Source: three-view drawing plus pictorial views. Frame: mm from the lowest corner of the part. A direction names the side the tool comes from. Round coordinates to 2 decimals unless told otherwise and drop trailing zeros. Write each loop counter-clockwise with the first axis right and the second up, starting at its lowest first coordinate (ties: lowest second). Pieces come first, ordered by that corner, then holes. Notation, with made-up numbers: (66.25, 66.25) -> (99.25, 66.25) arc R14 cw to (99.25, 74.25) -> close; hole circle Ø8 at (13, -12.5). An arc over 180 degrees is marked (long way). Put each result on its own line as item: value.
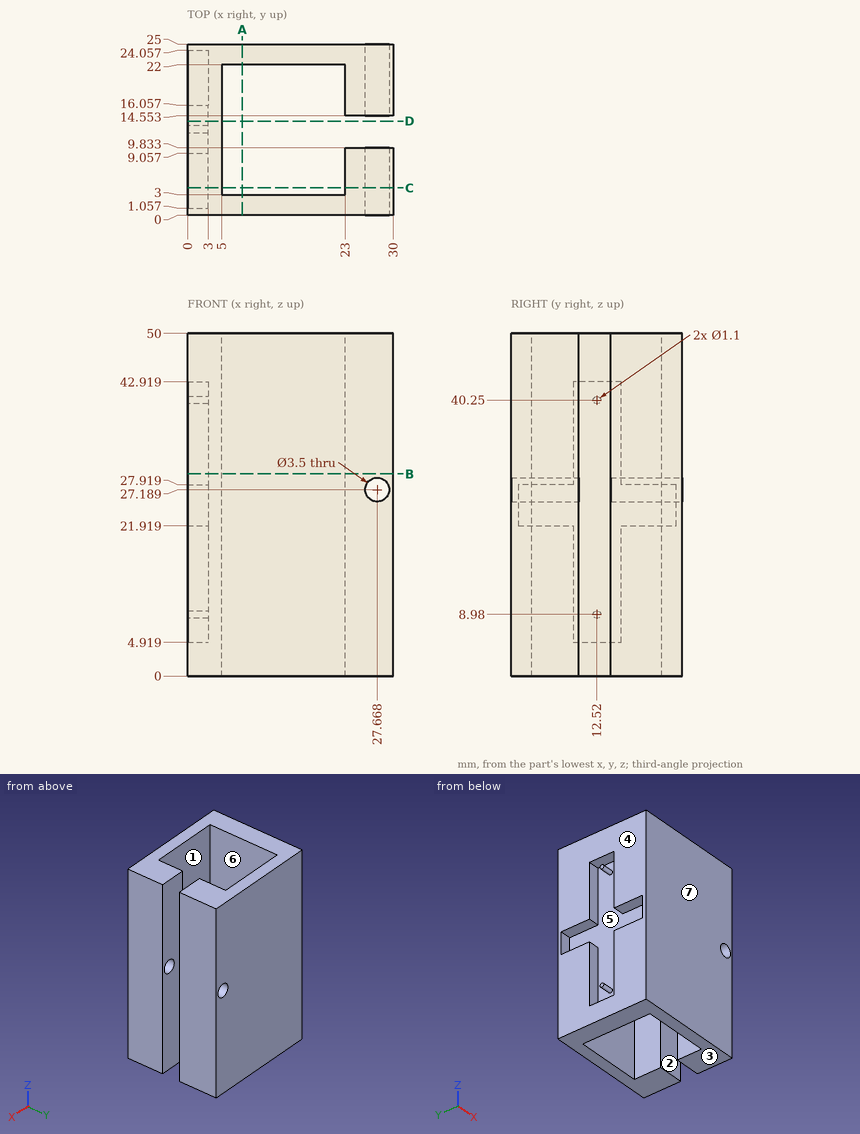
Q1. Material intervals for line 1 (Y direction, x = 2.75, z = 39.5); line 2 (X direction, y = 20.25, z = 42.5); line 3 (Y direction, x = 15.5, z = 33.5), sorted ascending. Write a range as [from, to].
Ans:
line 1: y = [0, 9.06], [16.06, 25]
line 2: x = [0, 5], [23, 30]
line 3: y = [0, 3], [22, 25]
Q2. Draft query along Y for the marked faces 4, 5, 6 and 7. Return one class per face: +Y half, -Y half, draft (parallel to the pull), parting line (faces both ways), or undercut.
Ans:
face 4: draft
face 5: undercut
face 6: undercut
face 7: -Y half
Q3. Cut plane A-A on x = 8. Output: boundary loops of the cut face in (y, z).
Ans:
outline: (0, 0) -> (3, 0) -> (3, 50) -> (0, 50) -> close; (22, 0) -> (25, 0) -> (25, 50) -> (22, 50) -> close
Q4. Reachability of the marked faces 1, 2 and 3 from +Z, -Z, +X, -X, +Y, -Y: full face, straight path, thin tool, end or side. Return the list, or none.
Ans:
face 1: +Z, -Z
face 2: +Z, -Z, +X
face 3: -Z, +X, -X, +Y, -Y
Q5. Cut plane D-D on y = 13.75. Output: boundary loops of the cut face in (x, z), and give its area (3 significant figures).
Ans:
outline: (0, 0) -> (5, 0) -> (5, 50) -> (0, 50) -> (0, 42.92) -> (3, 42.92) -> (3, 4.92) -> (0, 4.92) -> close
area: 136 mm^2
Q6. Cut plane C-C on y = 4. Output: boundary loops of the cut face in (x, z).
Ans:
outline: (0, 0) -> (5, 0) -> (5, 50) -> (0, 50) -> (0, 27.92) -> (3, 27.92) -> (3, 21.92) -> (0, 21.92) -> close; (23, 0) -> (30, 0) -> (30, 50) -> (23, 50) -> close; hole circle Ø3.5 at (27.67, 27.19)
Q7. Cut plane B-B on z = 29.5. Output: boundary loops of the cut face in (x, y), and give its area (3 significant figures).
Ans:
outline: (0, 0) -> (30, 0) -> (30, 9.83) -> (23, 9.83) -> (23, 3) -> (5, 3) -> (5, 22) -> (23, 22) -> (23, 14.55) -> (30, 14.55) -> (30, 25) -> (0, 25) -> (0, 16.06) -> (3, 16.06) -> (3, 9.06) -> (0, 9.06) -> close
area: 354 mm^2
